from build123d import *

# Parameters (mm, degrees)
SKETCH1_R                = 12.702118755
BOSS_EXTRUDE1_DEPTH      = 15
SKETCH1_3_R              = 5
CUT_EXTRUDE1_DEPTH       = 6
CUT_EXTRUDE3_DEPTH       = 81.715549927
CUT_EXTRUDE3_DEPTH_BACK  = 81.715549927
SKETCH1_4_R              = 2.05
FILLET1_R                = 10
CUT_EXTRUDE12_DEPTH      = 81.715550074
CUT_EXTRUDE12_DEPTH_BACK = 2.75
CUT_EXTRUDE12_START      = -7.5
SKETCH3_W                = 5.5
SKETCH3_H                = 2.5
CUT_EXTRUDE13_DEPTH      = 31.5
CUT_EXTRUDE14_DEPTH      = 21.5
CUT_EXTRUDE15_DEPTH      = 97.943282542
CUT_EXTRUDE15_DEPTH_BACK = 97.943282542
SKETCH4_R                = 5
FILLET2_R                = 5
CUT_EXTRUDE17_START      = -2.5
SKETCH6_R                = 2.05
SKETCH6_R_2              = 12.702118755
CUT_EXTRUDE17_DEPTH      = 2.5


with BuildPart() as part:
    # Sketch1 → Boss-Extrude1 (new body)
    with BuildSketch(Plane(origin=(0, 0, 0), x_dir=(0, 1, 0), z_dir=(0, 0, 1))):
        with BuildLine():
            Line((0, 31), (0, -31))
            Line((0, -31), (42, -31))
            ThreePointArc((42, -31), (73, 0), (42, 31))
            Line((42, 31), (0, 31))
        make_face()
        with Locations(Location((42, 0, 0), (0, 0, 270))):
            Circle(SKETCH1_R, mode=Mode.SUBTRACT)
    extrude(amount=BOSS_EXTRUDE1_DEPTH)

    # Sketch1<3> → Cut-Extrude1 (cut)
    with BuildSketch(Plane(origin=(0, 0, 0), x_dir=(0, 1, 0), z_dir=(0, 0, 1))):
        with Locations((59.5, 0)):
            Circle(SKETCH1_3_R)
        with Locations((42, -17.5)):
            Circle(SKETCH1_3_R)
        with Locations((24.5, 0)):
            Circle(SKETCH1_3_R)
        with Locations((42, 17.5)):
            Circle(SKETCH1_3_R)
    extrude(amount=CUT_EXTRUDE1_DEPTH, mode=Mode.SUBTRACT)

    # Sketch1<4> → Cut-Extrude3 (cut, two sides: drawn at the far end of the back side and taken through both)
    with BuildSketch(Plane(origin=(0, 0, 0), x_dir=(0, 1, 0), z_dir=(0, 0, 1)).offset(-CUT_EXTRUDE3_DEPTH_BACK)):
        with Locations(Location((59.5, 0, 0), (0, 0, 270))):
            Circle(SKETCH1_4_R)
        with Locations(Location((42, -17.5, 0), (0, 0, 270))):
            Circle(SKETCH1_4_R)
        with Locations(Location((24.5, 0, 0), (0, 0, 270))):
            Circle(SKETCH1_4_R)
        with Locations(Location((42, 17.5, 0), (0, 0, 270))):
            Circle(SKETCH1_4_R)
    extrude(amount=CUT_EXTRUDE3_DEPTH + CUT_EXTRUDE3_DEPTH_BACK, mode=Mode.SUBTRACT)

    # Fillet1
    fillet1_edges = [part.edges().sort_by_distance(p)[0] for p in [
        (-1.197579289, 29.354462261, 3),
        (1.197579289, 29.354462261, 3),
        (-12.645537739, 43.197579289, 3),
        (-12.645537739, 40.802420711, 3),
        (1.197579289, 54.645537739, 3),
        (-1.197579289, 54.645537739, 3),
        (12.645537739, 40.802420711, 3),
        (12.645537739, 43.197579289, 3),
    ]]
    fillet(fillet1_edges, radius=FILLET1_R)

    # Sketch3 → Cut-Extrude12 (cut, two sides: drawn at the far end of the back side and taken through both)
    with BuildSketch(Plane.XY.offset(15).offset(CUT_EXTRUDE12_START - CUT_EXTRUDE12_DEPTH_BACK)):
        with Locations((-23.25, 29.25)):
            Rectangle(SKETCH3_W, SKETCH3_H)
        with Locations((-7.75, 19.25)):
            Rectangle(SKETCH3_W, SKETCH3_H)
        with Locations((7.75, 19.25)):
            Rectangle(SKETCH3_W, SKETCH3_H)
        with Locations((23.25, 29.25)):
            Rectangle(SKETCH3_W, SKETCH3_H)
    extrude(amount=CUT_EXTRUDE12_DEPTH + CUT_EXTRUDE12_DEPTH_BACK, mode=Mode.SUBTRACT)

    # Sketch2 → Cut-Extrude13 (cut)
    with BuildSketch(Plane.XZ):
        with BuildLine():
            Line((-22.332277702, 6.189356729), (-23.25, 5.546760658))
            Line((-23.25, 5.546760658), (-24.167722298, 6.189356729))
            ThreePointArc((-24.167722298, 6.189356729), (-23.25, 9.1), (-22.332277702, 6.189356729))
        make_face()
        with BuildLine():
            Line((22.332277702, 6.189356729), (23.25, 5.546760658))
            Line((23.25, 5.546760658), (24.167722298, 6.189356729))
            ThreePointArc((24.167722298, 6.189356729), (23.25, 9.1), (22.332277702, 6.189356729))
        make_face()
    extrude(amount=-CUT_EXTRUDE13_DEPTH, mode=Mode.SUBTRACT)

    # Sketch2<3> → Cut-Extrude14 (cut)
    with BuildSketch(Plane.XZ):
        with BuildLine():
            Line((-8.667722298, 6.189356729), (-7.75, 5.546760658))
            Line((-7.75, 5.546760658), (-6.832277702, 6.189356729))
            ThreePointArc((-6.832277702, 6.189356729), (-7.75, 9.1), (-8.667722298, 6.189356729))
        make_face()
        with BuildLine():
            Line((6.832277702, 6.189356729), (7.75, 5.546760658))
            Line((7.75, 5.546760658), (8.667722298, 6.189356729))
            ThreePointArc((8.667722298, 6.189356729), (7.75, 9.1), (6.832277702, 6.189356729))
        make_face()
    extrude(amount=-CUT_EXTRUDE14_DEPTH, mode=Mode.SUBTRACT)

    # Sketch4 → Cut-Extrude15 (cut, two sides: drawn at the far end of the back side and taken through both)
    with BuildSketch(Plane(origin=(-31, 0, 0), x_dir=(0, -1, 0), z_dir=(-1, 0, 0)).offset(-CUT_EXTRUDE15_DEPTH_BACK)):
        with Locations((-42, -0.1)):
            Circle(SKETCH4_R)
    extrude(amount=CUT_EXTRUDE15_DEPTH + CUT_EXTRUDE15_DEPTH_BACK, mode=Mode.SUBTRACT)

    # Fillet2
    # the kernel refuses this fillet: 5 mm, written as the material it takes off along each edge
    with BuildSketch(Plane(origin=(-8.593139727, 37.0010001, 0), x_dir=(0, 0.2740416493582673, 0.9617178247370693), z_dir=(-1, 0, 0)), Plane(origin=(40.006860273, 37.0010001, 0), x_dir=(0, 0.2740416493582673, 0.9617178247370693), z_dir=(-1, 0, 0))) as fillet2_piece_1:
        with BuildLine():
            CenterArc((3.821287186, -4.835031475), FILLET2_R, 104.758918872, 59.336170258)
            Line((-0.987301938, -3.464823228), (0, 0))
            ThreePointArc((0, 0), (1.273762395, -0.164968525), (2.547524791, 0))
        make_face()
    extrude(amount=31.413720546, mode=Mode.SUBTRACT)
    with BuildSketch(Plane(origin=(-8.593139727, 46.9989999, 0), x_dir=(0, 1, 0), z_dir=(-1, 0, 0)), Plane(origin=(39.601140784, 46.9989999, 0), x_dir=(0, 1, 0), z_dir=(-1, 0, 0))) as fillet2_piece_2:
        with BuildLine():
            CenterArc((3.602744109, -5), FILLET2_R, 90, 59.336170258)
            ThreePointArc((-0.698127895, -2.45), (-0.190410776, -1.270208247), (0, 0))
            Line((0, 0), (3.602744109, 0))
        make_face()
    extrude(amount=31.008001057, mode=Mode.SUBTRACT)

    # Sketch6 → Cut-Extrude17 (cut)
    with BuildSketch(Plane.XY.offset(15).offset(CUT_EXTRUDE17_START)):
        with BuildLine():
            Line((-7.62767837, 21.898544265), (-6.15, 20.5))
            Line((-6.15, 20.5), (-5, 20.5))
            Line((-5, 20.5), (-5, 21.089476334))
            ThreePointArc((-5, 21.089476334), (0, 20.5), (5, 21.089476334))
            Line((5, 21.089476334), (5, 20.5))
            Line((5, 20.5), (6.15, 20.5))
            Line((6.15, 20.5), (7.389699175, 21.809845318))
            ThreePointArc((7.389699175, 21.809845318), (0.126985826, 63.499624987), (-7.62767837, 21.898544265))
        make_face()
        with Locations((0, 59.5)):
            Circle(SKETCH6_R, mode=Mode.SUBTRACT)
        with Locations((0, 24.5)):
            Circle(SKETCH6_R, mode=Mode.SUBTRACT)
        with Locations((-17.5, 42)):
            Circle(SKETCH6_R, mode=Mode.SUBTRACT)
        with Locations(Location((0, 42, 0), (0, 0, 221.332642507))):
            Circle(SKETCH6_R_2, mode=Mode.SUBTRACT)
        with Locations((17.5, 42)):
            Circle(SKETCH6_R, mode=Mode.SUBTRACT)
    extrude(amount=CUT_EXTRUDE17_DEPTH, mode=Mode.SUBTRACT)


solid = part.part
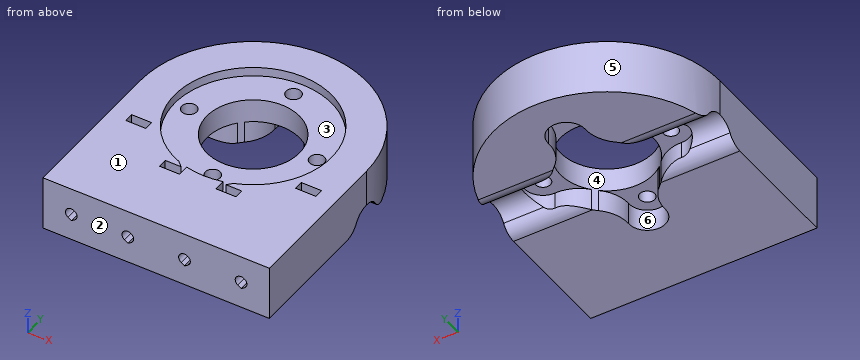
Build history of the part. All positions in model axes, mm. Face numbers are marked on the shaded views. A direction names the side the tool comes from. Coordinates: 2 decimals unless noted, no trailing zeros. Write each loop counter-clockwise with the first axis right and the second up, starting at its lowest first coordinate (ties: lowest second). Pieces come first, ordered by that corner, then holes. Notation, with made-up numbers: (-30.5, 88) -> (4.5, 88) arc R16 ccw to (4.5, 94) -> close; hole circle Ø4 at (40, 56.25). An arc over 180 degrees is marked (long way). Use CSV: the item, a comma, the result in double quotes. Start each with the question number.
Q1. 3-axis set-ups, long thin cutter, end or side, ignore diameter. For the marked faces 5 and 6: which of +Z, -Z, +X, -X, +Y, -Y reach the whole face in a straight line?
Q2. Flat gauge pins, fed straight in: pin 1 Ø4 at (x, z) = (-7.75, 7.5) entering from -Y; pin 2 Ø6.5 at (x, y) = (-2, 28) entering from -Z; pin 3 Ø3 at (x, z) = (21.5, 6) entering from +Y; pin 4 Ø1.5 at (y, z) = (63.5, 13.5) entering from -X. Where does each tip first touch, or does it go through?
Q3. Drill centre lines: probe 1 along X at (y, z) = (42, 7.5); probe 2 along Y at (x, z) = (0, 10.5); probe 3 along X at (y, z) = (4, 7.5). Where is each one in solid material? Low to high.
Q4. Pull direction Y, two halves, no side cores. Call the marked faces 1, 2, 3 and 4: released by +Y, released by -Y, zero draft, split by the parting line, or undercut.
Q5. Cut at A-A, the plane x = 0. List the corners of the cut face in (y, z), then the cut area to 3 significant figures.
Q6. Cut at B-B, the plane z = 7.5. State how many separate pieces and enclosed holes the cut face has, then the cut area to 3 significant figures.
Checked values:
1,face 5,"+Z, -Z, +Y"
1,face 6,"-Z"
2,pin 1,"stops at y = 0"
2,pin 2,"stops at z = 6"
2,pin 3,"stops at y = 65.69"
2,pin 4,"stops at x = -23.03"
3,probe 1,"x = -31 to -19.55, -15.45 to -12.7, 12.7 to 15.45, 19.55 to 31"
3,probe 2,"y = 0 to 22.45, 26.55 to 29.3, 54.7 to 57.45, 61.55 to 73"
3,probe 3,"x = -31 to -24.85, -21.65 to -9.35, -6.15 to 6.15, 9.35 to 21.65, 24.85 to 31"
4,face 1,"zero draft"
4,face 2,"released by -Y"
4,face 3,"undercut"
4,face 4,"undercut"
5,outline,"(0, 0) -> (19.5, 0) -> (19.5, 6) -> (22.45, 6) -> (22.45, 12.5) -> (20.5, 12.5) -> (20.5, 15) -> (0, 15) -> close; (26.55, 6) -> (29.3, 6) -> (29.3, 12.5) -> (26.55, 12.5) -> close; (54.7, 6) -> (57.45, 6) -> (57.45, 12.5) -> (54.7, 12.5) -> close; (61.55, 6) -> (64.5, 6) -> (64.5, 0) -> (73, 0) -> (73, 15) -> (63.5, 15) -> (63.5, 12.5) -> (61.55, 12.5) -> close"
5,area,"499 mm²"
6,separate pieces,"1"
6,enclosed holes,"5"
6,area,"3,190 mm²"
